```python
from build123d import *

# Parameters (mm, degrees)
SKETCH1_W           = 32
SKETCH1_H           = 32
BOSS_EXTRUDE1_DEPTH = 1.5
SKETCH3_W           = 17
SKETCH3_H           = 17
BOSS_EXTRUDE2_DEPTH = 2.5
SKETCH4_R           = 8
BOSS_EXTRUDE3_DEPTH = 12.5
SKETCH5_R           = 7.277770315
BOSS_EXTRUDE4_DEPTH = 2
SKETCH6_R           = 4
CUT_EXTRUDE1_DEPTH  = 2
CHAMFER1_SIZE       = 2
CHAMFER1_SIZE2      = 1.063418863
FILLET2_R           = 0.5


with BuildPart() as part:
    # Sketch1 → Boss-Extrude1 (new body)
    with BuildSketch(Plane.XY):
        Rectangle(SKETCH1_W, SKETCH1_H)
    extrude(amount=BOSS_EXTRUDE1_DEPTH)

    # Sketch3 → Boss-Extrude2 (add)
    with BuildSketch(Plane.XY.offset(1.5)):
        Rectangle(SKETCH3_W, SKETCH3_H)
    extrude(amount=BOSS_EXTRUDE2_DEPTH)

    # Sketch4 → Boss-Extrude3 (add)
    with BuildSketch(Plane.XY.offset(4)):
        with Locations(Location((0, 0, 0), (0, 0, 180))):
            Circle(SKETCH4_R)
    extrude(amount=BOSS_EXTRUDE3_DEPTH)

    # Sketch5 → Boss-Extrude4 (add)
    with BuildSketch(Plane.XY.offset(16.5)):
        Circle(SKETCH5_R)
    extrude(amount=BOSS_EXTRUDE4_DEPTH)

    # Sketch6 → Cut-Extrude1 (cut)
    with BuildSketch(Plane.XY.offset(18.5)):
        Circle(SKETCH6_R)
    extrude(amount=-CUT_EXTRUDE1_DEPTH, mode=Mode.SUBTRACT)

    # Chamfer1
    chamfer1_edges = [part.edges().sort_by_distance(p)[0] for p in [
        (-4, 0, 18.5),
    ]]
    chamfer1_side = [part.faces().sort_by_distance(p)[0] for p in [
        (-7.071923885, 0, 18.5),
    ]]
    chamfer(chamfer1_edges, length=CHAMFER1_SIZE, length2=CHAMFER1_SIZE2, reference=chamfer1_side[0])

    # Fillet2
    fillet2_edges = [part.edges().sort_by_distance(p)[0] for p in [
        (8.5, 0, 4),
        (0, 8.5, 4),
        (-8.5, 0, 4),
        (0, -8.5, 4),
    ]]
    fillet(fillet2_edges, radius=FILLET2_R - 0.0001)  # a hair under: the kernel refuses the full size


solid = part.part
```
Geometry check sheet. Reference: the model listing, model coordinates, mm. A direction names the side the tool comes from. Give positions to 0.01 mm unless a question says otherwise; leave off trailing zeros. Order: outer loops, then holes, each group sorted by start corner. A loop starts at its lowest first (then second) coordinate and runs counter-clockwise, first axis right, second up.
1. Access from +Z, -Z, +X, -X, +Y, -Y to the whole of each face (thin tool, end or side, straight path). Record for faces 4 (the face through (-8.5, 0, 2)), 5 (the face through (1.73, 7.81, 10.16)), 6 (the face through (0, 8.5, 2)), 7 (the face through (0, -8.5, 2)), 8 (the face through (8.5, 0, 2)).
2. Section check C-C, the plane y = -11.5. Enter the section's corners in (x, z).
3. Gauge pin test, flat ends, axial feed: pin 1 Ø2.5 at (x, y) = (-0.5, 0) entering from +Z; pin 2 Ø0.6 at (y, z) = (2.5, 2.5) entering from -X; pin 3 Ø1 at (x, y) = (-9.5, -4.5) entering from +Z. Record the tip position at first contact, or that the pin passes through.
4. Section check D-D, the plane x = -6.5. Enter the section's corners in (y, z), and give its area (3 significant figures).
5. Release check for a two-part mould opening along X. For faces 1 (the face through (-5.364, 4.919, 17.486)), 2 (the face through (0, 0, 0)), 3 (the face through (0, 0, 16.5)) record: pulls with the +X half, pulls with the -X half, needs draft (parallel to the pull), parting line crosses it, or undercut.
6. Thickness scan on L1, parallel to Y at x = 0, z = 16.7; L2, parallel to Z at x = -14, y = 9.5; L3, parallel to Z at x = 7.5, y = -0.5. Record the ranges inside material, lowest first.
Values follow:
1. face 4: +Z, -X, +Y, -Y
1. face 5: +Z
1. face 6: +Z, +X, -X, +Y
1. face 7: +Z, +X, -X, -Y
1. face 8: +Z, +X, +Y, -Y
2. outline: (-16, 0) - (16, 0) - (16, 1.5) - (-16, 1.5) - close
3. pin 1: stops at z = 16.5
3. pin 2: stops at x = -8.5
3. pin 3: stops at z = 1.5
4. outline: (-16, 0) - (16, 0) - (16, 1.5) - (8.5, 1.5) - (8.5, 3.5) arc R0.5 ccw to (8, 4) - (4.66, 4) - (4.66, 16.5) - (3.27, 16.5) - (3.27, 18.5) - (-3.27, 18.5) - (-3.27, 16.5) - (-4.66, 16.5) - (-4.66, 4) - (-8, 4) arc R0.5 ccw to (-8.5, 3.5) - (-8.5, 1.5) - (-16, 1.5) - close
4. area: 220 mm2
5. face 1: parting line crosses it
5. face 2: needs draft
5. face 3: undercut
6. L1: y = -7.28 to -4, 4 to 7.28
6. L2: z = 0 to 1.5
6. L3: z = 0 to 16.5
